Could you check a few things on this model? Use its own coordinates, in mm. A direction names the side the tool comes from. Coordinates: 2 decimals unless noted, no trailing zeros. Loops run counter-clockwise (first coordinate to the right, second up) from the corner with the lowest first, then second, coordinate; pieces in that order, holes last.
from build123d import *

# Parameters (mm, degrees)
BOX021_W     = 4.5
BOX021_H     = 1
BOX021_DEPTH = 1
BOX020_W     = 4.5
BOX020_H     = 1
BOX020_DEPTH = 1
BOX019_W     = 14
BOX019_H     = 14
BOX019_DEPTH = 5.2
BOX018_W     = 24
BOX018_H     = 24
BOX018_DEPTH = 5.2


with BuildPart() as slot_top001:
    # Box021 → Box021 (new body)
    with BuildSketch(Plane(origin=(9.75, 19, -2.2), x_dir=(1, 0, 0), z_dir=(0, 0, 1))):
        with Locations((2.25, 0.5)):
            Rectangle(BOX021_W, BOX021_H)
    extrude(amount=BOX021_DEPTH)


with BuildPart() as slot_bottom001:
    # Box020 → Box020 (new body)
    with BuildSketch(Plane(origin=(9.75, 4, -2.2), x_dir=(1, 0, 0), z_dir=(0, 0, 1))):
        with Locations((2.25, 0.5)):
            Rectangle(BOX020_W, BOX020_H)
    extrude(amount=BOX020_DEPTH)


with BuildPart() as cutout001:
    # Box019 → Box019 (new body)
    with BuildSketch(Plane(origin=(5, 5, 0), x_dir=(1, 0, 0), z_dir=(0, 0, 1))):
        with Locations((7, 7)):
            Rectangle(BOX019_W, BOX019_H)
    extrude(amount=BOX019_DEPTH)


with BuildPart() as cut009:
    # Box018 → Box018 (new body)
    with BuildSketch(Plane.XY):
        with Locations((12, 12)):
            Rectangle(BOX018_W, BOX018_H)
    extrude(amount=BOX018_DEPTH)

    # Cut007: cut CutOut001
    add(cutout001.part, mode=Mode.SUBTRACT)


with BuildPart() as cut009_1:
    # Cut007 placement: moved
    add(cut009.part.moved(Location((0, 0, -5.2))))

    # Cut008: cut slot_bottom001
    add(slot_bottom001.part, mode=Mode.SUBTRACT)

    # Cut009: cut slot_top001
    add(slot_top001.part, mode=Mode.SUBTRACT)


solid = cut009_1.part
(1) Imagine slicing it at A-A, the plane z = -4.6. Write out the boundary of the cut face in (x, y).
Answers:
outline: (0, 0) - (24, 0) - (24, 24) - (0, 24) - close; hole (5, 5) - (19, 5) - (19, 19) - (5, 19) - close
(2) We'd pull the mould along X, two halves only. Please class faces 4 (the face through (4, 12, 0)), 5 (the face through (0, 12, -3)), 6 (the face through (19, 12, -3)): +X half, -X half, draft (parallel to the pull), parting line (faces both ways), or undercut.
Answers:
face 4: draft
face 5: -X half
face 6: undercut
(3) Imagine slicing it at B-B, the plane y = 13. Write out the boundary of the cut face in (x, z).
Answers:
outline: (0, -5.2) - (5, -5.2) - (5, 0) - (0, 0) - close; (19, -5.2) - (24, -5.2) - (24, 0) - (19, 0) - close
(4) Which directions (+Z, -Z, +X, -X, +Y, -Y) give clear straight access to the entire face, cutting with the end or side of a thin tool? Please do faces 1 (the face through (4, 12, -5.2)), 2 (the face through (12, 4, -2)), 3 (the face through (12, 5, -3)).
Answers:
face 1: -Z, +X, -X, +Y, -Y
face 2: none
face 3: +Z, -Z
(5) For pin 1 (8 mm diameter, centred on x = 9.5, y = 14, fed in from +Z), with a flat end and sliding along its axis, tell me the tip position at first contact or that it passes through.
Answers:
pin 1: passes through
(6) I need wall thicknesses on probe 1 along Y at (x, z) = (7, -0.35). Which ranges of the line are inside material? Lowest first, please.
Answers:
probe 1: y = 0 to 5, 19 to 24
(7) Imagine slicing it at C-C, the plane x = 10.25. Write out the boundary of the cut face in (y, z).
Answers:
outline: (0, -5.2) - (5, -5.2) - (5, -2.2) - (4, -2.2) - (4, -1.2) - (5, -1.2) - (5, 0) - (0, 0) - close; (19, -5.2) - (24, -5.2) - (24, 0) - (19, 0) - (19, -1.2) - (20, -1.2) - (20, -2.2) - (19, -2.2) - close
